Geometry: final body of the model. Coordinates: model frame, mm. Face numbers are marked on the shaded views. Give positions to 0.01 mm unless a question says otherwise; leave off trailing zeros. Write each loop counter-clockwise with the first axis right and the second up, starting at its lowest first coordinate (ties: lowest second). Pieces come first, ordered by that corner, then holes.
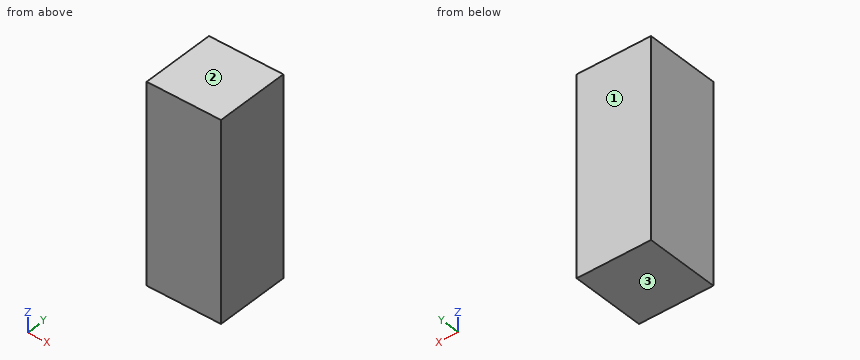
```python
from build123d import *

# Parameters (mm, degrees)
SKETCH1_W           = 15
SKETCH1_H           = 15
BOSS_EXTRUDE1_DEPTH = 20
SKETCH2_R           = 5
CUT_EXTRUDE1_DEPTH  = 17.5


with BuildPart() as part:
    # Sketch1 → Boss-Extrude1 (new body, symmetric)
    with BuildSketch(Plane.XY):
        Rectangle(SKETCH1_W, SKETCH1_H)
    extrude(amount=BOSS_EXTRUDE1_DEPTH, both=True)

    # Sketch2 → Cut-Extrude1 (cut, symmetric)
    with BuildSketch(Plane.XY):
        Circle(SKETCH2_R)
    extrude(amount=CUT_EXTRUDE1_DEPTH, both=True, mode=Mode.SUBTRACT)


solid = part.part
```
Item 1: Line query: L1, parallel to Z at x = -3.75, y = 2; L2, parallel to Y at x = 0, z = -6.5; L3, parallel to Y at x = 1, z = 0. Output: solid intervals per line, ascending.
Found:
L1: z = -20 to -17.5, 17.5 to 20
L2: y = -7.5 to -5, 5 to 7.5
L3: y = -7.5 to -4.9, 4.9 to 7.5
Item 2: Pull-direction query (Z, two-part tool) for the marked faces 1, 2 and 3; classes: +Z half, -Z half, draft (parallel to the pull), parting line (faces both ways), or undercut.
Found:
face 1: draft
face 2: +Z half
face 3: -Z half
Item 3: Section C-C, the plane y = 0. Return the cut outline in (x, z).
Found:
outline: (-7.5, -20) - (7.5, -20) - (7.5, 20) - (-7.5, 20) - close; hole (-5, -17.5) - (5, -17.5) - (5, 17.5) - (-5, 17.5) - close
Item 4: Section B-B, the plane z = 17. Return the cut outline in (x, y).
Found:
outline: (-7.5, -7.5) - (7.5, -7.5) - (7.5, 7.5) - (-7.5, 7.5) - close; hole circle Ø10 at (0, 0)
Item 5: Section A-A, the plane x = 3. Return the cut outline in (y, z).
Found:
outline: (-7.5, -20) - (7.5, -20) - (7.5, 20) - (-7.5, 20) - close; hole (-4, -17.5) - (4, -17.5) - (4, 17.5) - (-4, 17.5) - close
